For this review, use the dimensioned drawing (mm, ordinates from the lowest corner) and the shaded views. Give positions to 0.01 mm unless a question says otherwise; leave off trailing zeros. Write each loop counter-clockwise with the first axis right and the second up, starting at its lowest first coordinate (ties: lowest second). Pieces come first, ordered by that corner, then holes.
1) We need section A-A on y = 12.7. Give the boundary of the cut face in (x, z) (1 decimal).
2) Wall thickness on line 1 along Y through (x, z) = (63.5, 1.65); line 2 along X through (y, z) = (14, 2.25) (1 decimal); line 3 along Y through (x, z) = (12.5, 1.55): over which ranges is each line inside the solid? List them lowest first.
3) We need section D-D on y = 38.1. Give the boundary of the cut face in (x, z) (1 decimal).
4) For P1, Ø0.9, axis at y = 42.5, z = 1.5, coming from the -X side; P2, Ø5.5, axis at x = 12.7, y = 12.7, coming from the -Z side; P3, Ø2, axis at x = 25, y = 12, coming from the -Z side; P4, Ø1.6, axis at x = 15.5, z = 2, coming from the +Y side, all flat-tipped, find the tip position at first contact; note any pin that passes through.
5) We need section C-C on z = 0.7. Give the number of separate pieces and of enclosed holes in the cut face, and give its area (3 significant figures).
6) We need section B-B on x = 25.4. Give the boundary of the cut face in (y, z) (1 decimal).
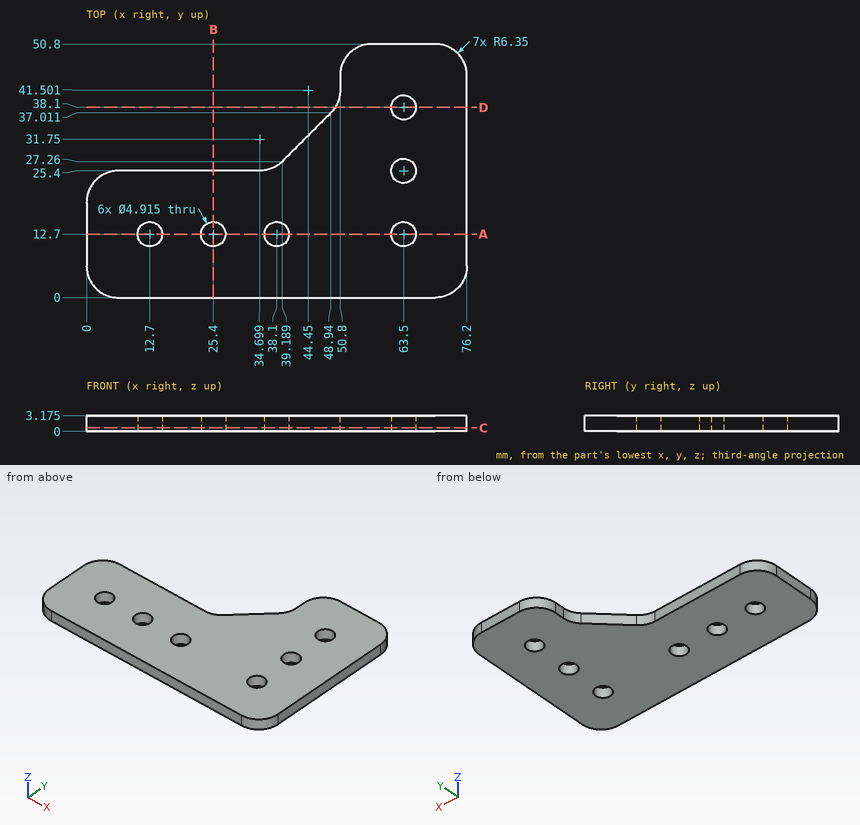
Results list:
1. outline: (0, 0) - (10.2, 0) - (10.2, 3.2) - (0, 3.2) - close; (15.2, 0) - (22.9, 0) - (22.9, 3.2) - (15.2, 3.2) - close; (27.9, 0) - (35.6, 0) - (35.6, 3.2) - (27.9, 3.2) - close; (40.6, 0) - (61, 0) - (61, 3.2) - (40.6, 3.2) - close; (66, 0) - (76.2, 0) - (76.2, 3.2) - (66, 3.2) - close
2. line 1: y = 0 to 10.24, 15.16 to 22.94, 27.86 to 35.64, 40.56 to 50.8
2. line 2: x = 0 to 10.6, 14.8 to 23.3, 27.5 to 36, 40.2 to 61.4, 65.6 to 76.2
2. line 3: y = 0 to 10.25, 15.15 to 25.4
3. outline: (49.8, 0) - (61, 0) - (61, 3.2) - (49.8, 3.2) - close; (66, 0) - (76.2, 0) - (76.2, 3.2) - (66, 3.2) - close
4. P1: stops at x = 50.8
4. P2: stops at z = 0
4. P3: passes through
4. P4: stops at y = 25.4
5. separate pieces: 1
5. enclosed holes: 6
5. area: 2,520 mm2
6. outline: (0, 0) - (10.2, 0) - (10.2, 3.2) - (0, 3.2) - close; (15.2, 0) - (25.4, 0) - (25.4, 3.2) - (15.2, 3.2) - close
